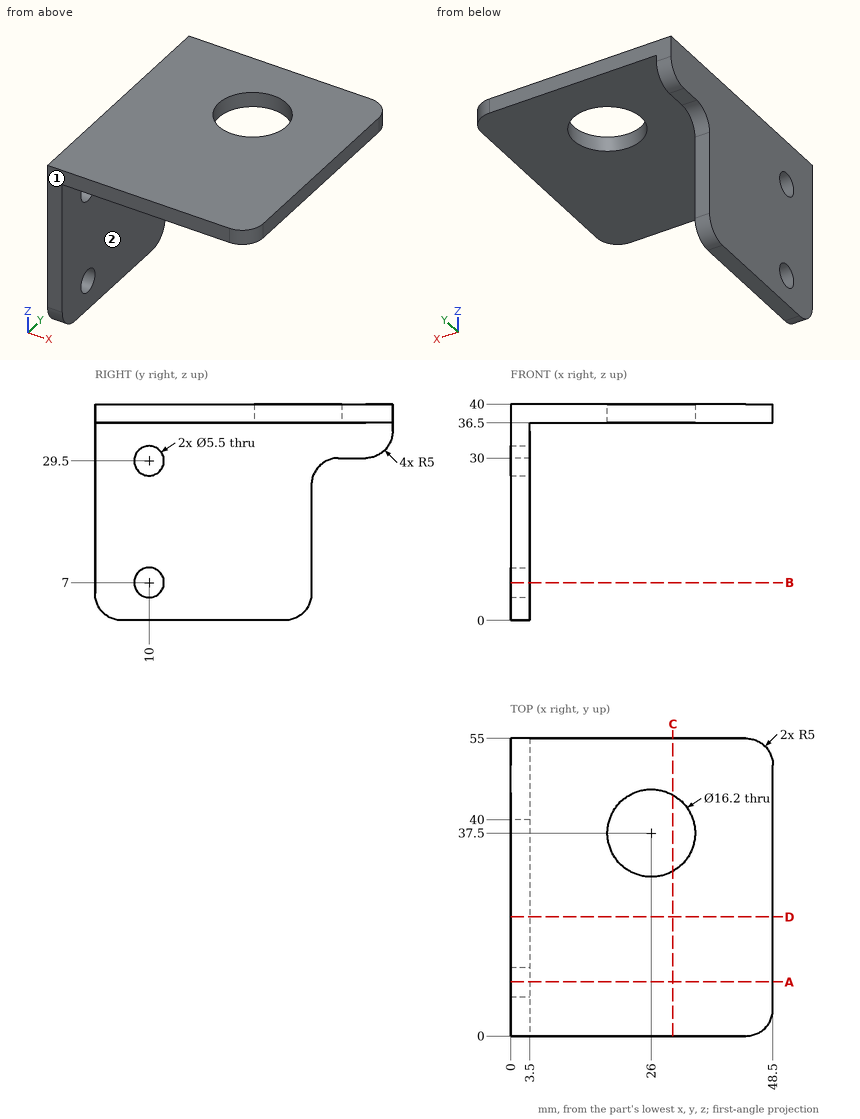
Source: three-view drawing plus pictorial views. Frame: mm from the lowest corner of the part. A direction names the side the tool comes from. Give positions to 0.01 mm unless a question says otherwise; leave off trailing zeros. Order: outer loops, then holes, each group sorted by start corner. A loop starts at its lowest first (then second) coordinate and runs counter-clockwise, first axis right, second up. Notation, with made-up numbers: (-24.75, 58) - (2.25, 58) arc R29 ccw to (2.25, 85) - close; hole circle Ø2 at (-18.5, -37.5). An arc over 180 degrees is marked (long way). Answer as a JSON object with one key per item and string values. Group by question number.
Q1. Line query: probe 1 along Y at (x, z) = (0.8, 7); probe 2 along X at (y, z) = (10.5, 20); probe 3 along Z at (x, y) = (11.5, 47.5). Output: solid intervals per line, ascending.
Q2. Cut plane D-D, the plane y = 22. Output: boundary loops of the cut face in (x, z).
Q3. Cut plane C-C, the plane x = 30. Output: boundary loops of the cut face in (y, z).
Q4. Set-up query: the marked faces 1 and 2. Return all of +Z, -Z, +X, -X, +Y, -Y with unobstructed straight access to the full face (end or side cutting, diameter ignored); none if empty.
Q5. Cut plane A-A, the plane y = 10. Output: boundary loops of the cut face in (x, z).
Q6. First-contact query: pin 1 Ø3.5 at (y, z) = (10, 7) entering from +X; pin 2 Ø4 at (y, z) = (6, 6) entering from +X; pin 3 Ø12 at (x, y) = (33.5, 8) entering from -Z; pin 4 Ø3 at (x, y) = (2, 47) entering from -Z. Flat tips, straight axial feed; report the tip coordinate or a pass-through.
Q7. Cut plane B-B, the plane z = 7. Output: boundary loops of the cut face in (x, y).
Results:
{
 "1": {"probe 1": "0 to 7.25, 12.75 to 40", "probe 2": "0 to 3.5", "probe 3": "36.5 to 40"},
 "2": {"outline": "(0, 0) - (3.5, 0) - (3.5, 36.5) - (48.5, 36.5) - (48.5, 40) - (0, 40) - close"},
 "3": {"outline": "(0, 36.5) - (30.46, 36.5) - (30.46, 40) - (0, 40) - close; (44.54, 36.5) - (55, 36.5) - (55, 40) - (44.54, 40) - close"},
 "4": {"face 1": "+Z, -Z, +X, -X, -Y", "face 2": "-Z, +X, +Y, -Y"},
 "5": {"outline": "(0, 0) - (3.5, 0) - (3.5, 4.25) - (0, 4.25) - close; (0, 9.75) - (3.5, 9.75) - (3.5, 26.75) - (0, 26.75) - close; (0, 32.25) - (3.5, 32.25) - (3.5, 36.5) - (48.5, 36.5) - (48.5, 40) - (0, 40) - close"},
 "6": {"pin 1": "through", "pin 2": "x = 3.5", "pin 3": "z = 36.5", "pin 4": "z = 30"},
 "7": {"outline": "(0, 0) - (3.5, 0) - (3.5, 7.25) - (0, 7.25) - close; (0, 12.75) - (3.5, 12.75) - (3.5, 40) - (0, 40) - close"}
}
